Geometry check sheet. Reference: the model listing, model coordinates, mm. Face numbers are marked on the shaded views. A direction names the side the tool comes from. Give positions to 0.01 mm unless a question says otherwise; leave off trailing zeros. Write each loop counter-clockwise with the first axis right and the second up, starting at its lowest first coordinate (ties: lowest second). Pieces come first, ordered by that corner, then holes.
(1) Cross-section at D-D (x = -9). Record the boundary of the cut face in (y, z).
(2) Tool access check on the marked faces 4, 5 and 6. Record the directions out of +Z, -Z, +X, -X, +Y, -Y that give a thin tool (end or side, any length) a straight path to the whole face; none if there is none.
(3) Cross-section at A-A (y = 0). Record the boundary of the cut face in (x, z) (3 decimals).
(4) Cross-section at C-C (x = 6). Record the boundary of the cut face in (y, z), and give its area (3 significant figures).
(5) Depth check by flat-ended pin: P1, Ø6, axis at x = 12, z = -8, coming from the -Y side; P2, Ø2, axis at x = -11, y = 8.5, coming from the -Z side; P3, Ø1, axis at x = 1.5, y = 2, coming from the -Z side. Enter the tip coordinate at first touch or a pass-through.
(6) Thickness scan on line 1 along X through (y, z) = (0, 8.95) (3 decimals); line 2 along Z through (x, y) = (2.5, -0.25); line 3 along Z through (x, y) = (11.5, 0). Record the ranges inside material, lowest first.
(7) Mould release check, pull along X, two halves, no side actions. Record for the marked faces 1, 2 and 3: +X half, -X half, draft (parallel to the pull), parting line (faces both ways), or undercut.
(8) Cross-section at B-B (z = 0). Record the boundary of the cut face in (x, y), and give its area (3 significant figures).
```python
from build123d import *

# Parameters (mm, degrees)
F0_R     = 11.176
F0_R_2   = 6
F1_DEPTH = 19.05
F2_R     = 11.176
F2_R_2   = 5
F3_DEPTH = 19.05
F4_SIZE  = 0.762
F7_D     = 5
F7_DEPTH = 12.7
F7_START = 0.2832054
F7_TIP   = 1.5021515476


with BuildPart() as f1:
    # F0 (on Right) → F1 (new body)
    with BuildSketch(Plane.YZ):
        Circle(F0_R)
        Circle(F0_R_2, mode=Mode.SUBTRACT)
    extrude(amount=-F1_DEPTH)

    # F2 (on Right) → F3 (join)
    with BuildSketch(Plane.YZ):
        Circle(F2_R)
        Circle(F2_R_2, mode=Mode.SUBTRACT)
    extrude(amount=F3_DEPTH)

    # F4
    f4_edges = [f1.edges().sort_by_distance(p)[0] for p in [
        (-19.05, -11.176, 0),
        (19.05, -11.176, 0),
    ]]
    chamfer(f4_edges, length=F4_SIZE)

    # F7
    # its depths count from where the whole tool has entered the part; down to there all is cleared
    with Locations(Plane.XY.offset(11.176).offset(-F7_START)):
        with Locations((-9.525, 0), (9.525, 0)):
            Hole(F7_D / 2, depth=F7_DEPTH)
            with Locations((0, 0, -(F7_DEPTH + F7_TIP / 2))):  # 118° drill point
                Cone(0, F7_D / 2, F7_TIP, mode=Mode.SUBTRACT)


solid = f1.part
```
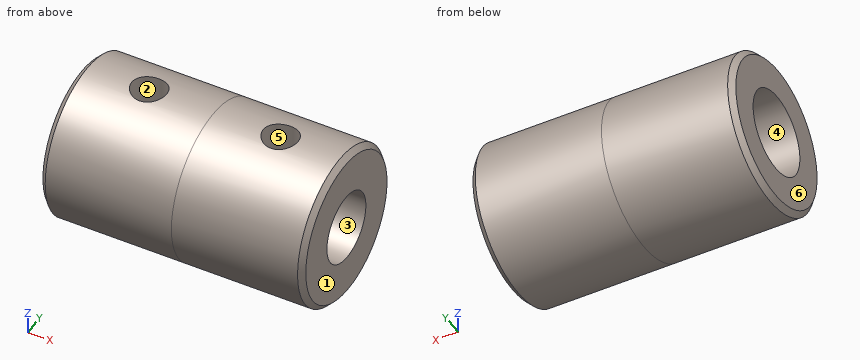
Reply:
1. outline: (-2.44, 5.48) - (-2.44, 10.91) arc R11.18 ccw (long way) to (2.44, 10.91) - (2.44, 5.48) arc R6 cw (long way) to start
2. face 4: -X
2. face 5: +Z
2. face 6: +Z, -Z, -X, +Y, -Y
3. outline: (-19.05, -10.414) - (-18.288, -11.176) - (18.288, -11.176) - (19.05, -10.414) - (19.05, -5) - (0, -5) - (0, -6) - (-19.05, -6) - close; (-19.05, 6) - (-12.025, 6) - (-12.025, 11.176) - (-18.288, 11.176) - (-19.05, 10.414) - close; (-7.025, 6) - (0, 6) - (0, 5) - (7.025, 5) - (7.025, 11.176) - (-7.025, 11.176) - close; (12.025, 5) - (19.05, 5) - (19.05, 10.414) - (18.288, 11.176) - (12.025, 11.176) - close
4. outline: circle Ø22.35 at (0, 0); hole circle Ø10 at (0, 0)
4. area: 314 mm2
5. P1: stops at y = -10
5. P2: stops at z = -8.29
5. P3: stops at z = -11.07
6. line 1: x = -19.05 to -12.025, -7.025 to 7.025, 12.025 to 19.05
6. line 2: z = -11.17 to -4.99, 4.99 to 11.17
6. line 3: z = -11.18 to -5
7. face 1: +X half
7. face 2: undercut
7. face 3: draft
8. outline: (-19.05, -10.41) - (-18.29, -11.18) - (18.29, -11.18) - (19.05, -10.41) - (19.05, -5) - (0, -5) - (0, -6) - (-19.05, -6) - close; (-19.05, 6) - (0, 6) - (0, 5) - (19.05, 5) - (19.05, 10.41) - (18.29, 11.18) - (-18.29, 11.18) - (-19.05, 10.41) - close
8. area: 431 mm2
